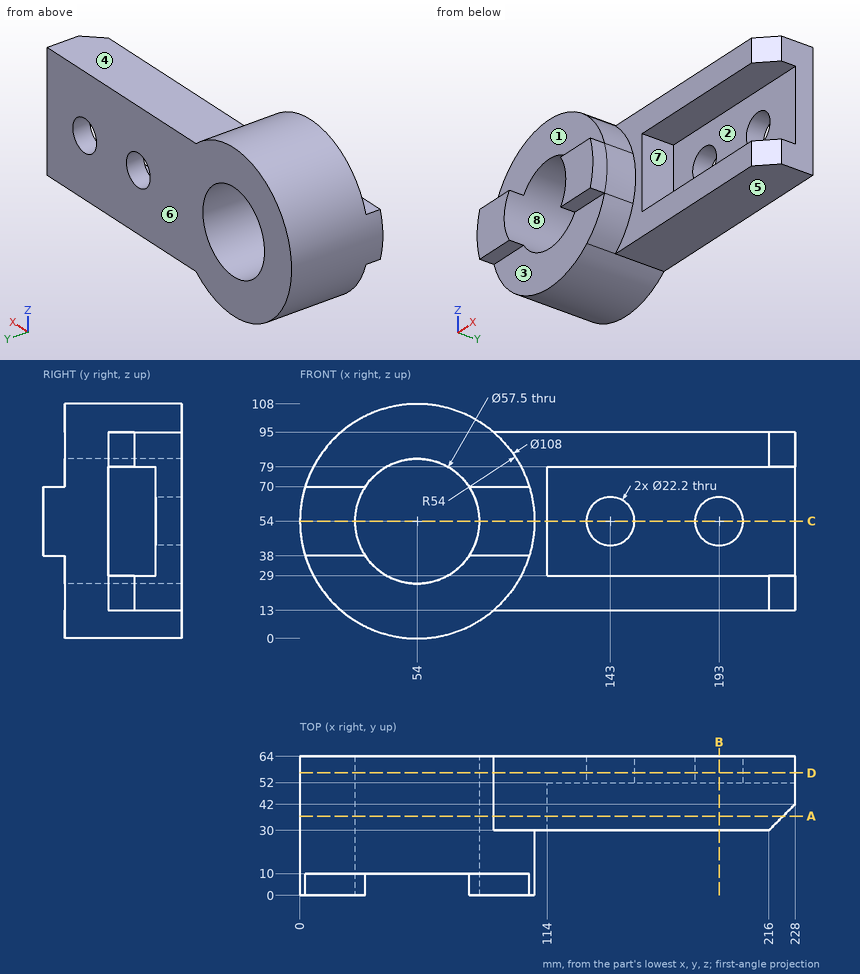
Print and shaded views of the part. All mm, measured from the part's lowest x, y and z. A direction names the side the tool comes from. Give positions to 0.01 mm unless a question says otherwise; leave off trailing zeros. Write each loop counter-clockwise with the first axis right and the second up, starting at its lowest first coordinate (ties: lowest second). Pieces come first, ordered by that corner, then holes. Notation, with made-up numbers: (-12, 68) - (-1, 68) arc R25 cw to (-1, 96) - close; hole circle Ø7 at (-12, -29.75). An arc over 180 degrees is marked (long way). One line per question, with ' | ' between items. Start each with the question number.
(1) Two-plate mould, pull along X, no slides. Class the marked faces 6, 7 and 8: +X half, -X half, draft (parallel to the pull), parting line (faces both ways), or undercut.
(2) Slice it at B-B on x = 193. Write the cut outline in (y, z), plus the area to 3 significant figures.
(3) Wall check: line 1 along Z through (x, y) = (143, 60); line 2 along X through (y, z) = (43, 54); line 3 along Z through (x, y) = (54, 33). Give the ranges that are in metal, low to high. Write a range as from..to.
(4) Slice it at A-A on y = 36.5. Write the cut outline in (x, z).
(5) Slice it at D-D on y = 56.5. Write the cut outline in (x, z).
(6) Slice it at C-C on z = 54. Write the cut outline in (x, y).
(7) Pin check, flat tips, straight feed: P1, Ø10, axis at x = 158.5, y = 54.5, coming from the -Z side; P2, Ø20, axis at x = 143, z = 54, coming from the +Y side; P3, Ø2, axis at y = 18, z = 60, coming from the +X side; P4, Ø8, axis at x = 142.5, z = 72, coming from the -Y side. Stop position of each tip, or through.
(8) 3-axis set-ups, long thin cutter, end or side, ignore diameter. For the marked faces 1, 2, 3, 4 and 5: which of +Z, -Z, +X, -X, +Y, -Y reach the whole face in a straight line?
Results below:
1) face 6: draft | face 7: +X half | face 8: undercut
2) outline: (30, 13) - (64, 13) - (64, 42.9) - (52, 42.9) - (52, 29) - (30, 29) - close; (30, 79) - (52, 79) - (52, 65.1) - (64, 65.1) - (64, 95) - (30, 95) - close | area: 1,420 mm^2
3) line 1: 13..42.9, 65.1..95 | line 2: 0..25.25, 82.75..114 | line 3: 0..25.25, 82.75..108
4) outline: (89.14, 13) - (222.5, 13) - (222.5, 29) - (114, 29) - (114, 79) - (222.5, 79) - (222.5, 95) - (89.14, 95) arc R54 ccw (long way) to start; hole circle Ø57.5 at (54, 54)
5) outline: (89.14, 13) - (228, 13) - (228, 95) - (89.14, 95) arc R54 ccw (long way) to start; hole circle Ø57.5 at (54, 54); hole circle Ø22.2 at (143, 54); hole circle Ø22.2 at (193, 54)
6) outline: (0, 0) - (25.25, 0) - (25.25, 64) - (0, 64) - close; (82.75, 0) - (108, 0) - (108, 30) - (114, 30) - (114, 52) - (131.9, 52) - (131.9, 64) - (82.75, 64) - close; (154.1, 52) - (181.9, 52) - (181.9, 64) - (154.1, 64) - close; (204.1, 52) - (228, 52) - (228, 64) - (204.1, 64) - close
7) P1: z = 13 | P2: through | P3: x = 107.77 | P4: y = 52
8) face 1: +Z, +X, -X, -Y | face 2: +X, -Y | face 3: -Z, +X, -X, -Y | face 4: +Z, +X, +Y, -Y | face 5: -Z, +X, +Y, -Y
